```python
from build123d import *

# Parameters (mm, degrees)
SKETCH1_R           = 0.75
BOSS_EXTRUDE1_DEPTH = 1.2


with BuildPart() as part:
    # Sketch1 → Boss-Extrude1 (new body)
    with BuildSketch(Plane.XY):
        with BuildLine():
            Line((13, 8.65), (-13, 8.65))
            Line((-13, 8.65), (-13, 7.6))
            ThreePointArc((-13, 7.6), (-12.469669914, 7.380330086), (-12.25, 6.85))
            ThreePointArc((-12.25, 6.85), (-12.469669914, 6.319669914), (-13, 6.1))
            Line((-13, 6.1), (-13, 5.4))
            ThreePointArc((-13, 5.4), (-12.469669914, 5.180330086), (-12.25, 4.65))
            ThreePointArc((-12.25, 4.65), (-12.469669914, 4.119669914), (-13, 3.9))
            Line((-13, 3.9), (-13, -3.9))
            ThreePointArc((-13, -3.9), (-12.469669914, -4.119669914), (-12.25, -4.65))
            ThreePointArc((-12.25, -4.65), (-12.469669914, -5.180330086), (-13, -5.4))
            Line((-13, -5.4), (-13, -6.1))
            ThreePointArc((-13, -6.1), (-12.469669914, -6.319669914), (-12.25, -6.85))
            ThreePointArc((-12.25, -6.85), (-12.469669914, -7.380330086), (-13, -7.6))
            Line((-13, -7.6), (-13, -8.65))
            Line((-13, -8.65), (13, -8.65))
            Line((13, -8.65), (13, -7.6))
            ThreePointArc((13, -7.6), (12.25, -6.85), (13, -6.1))
            Line((13, -6.1), (13, -5.4))
            ThreePointArc((13, -5.4), (12.25, -4.65), (13, -3.9))
            Line((13, -3.9), (13, 3.9))
            ThreePointArc((13, 3.9), (12.25, 4.65), (13, 5.4))
            Line((13, 5.4), (13, 6.1))
            ThreePointArc((13, 6.1), (12.25, 6.85), (13, 7.6))
            Line((13, 7.6), (13, 8.65))
        make_face()
        with Locations((-11.3, -6.85)):
            Circle(SKETCH1_R, mode=Mode.SUBTRACT)
        with Locations((-11.3, -4.65)):
            Circle(SKETCH1_R, mode=Mode.SUBTRACT)
        with Locations((11.3, -6.85)):
            Circle(SKETCH1_R, mode=Mode.SUBTRACT)
        with Locations((11.3, -4.65)):
            Circle(SKETCH1_R, mode=Mode.SUBTRACT)
        with Locations((-11.3, 4.65)):
            Circle(SKETCH1_R, mode=Mode.SUBTRACT)
        with Locations((-11.3, 6.85)):
            Circle(SKETCH1_R, mode=Mode.SUBTRACT)
        with Locations((11.3, 4.65)):
            Circle(SKETCH1_R, mode=Mode.SUBTRACT)
        with Locations((11.3, 6.85)):
            Circle(SKETCH1_R, mode=Mode.SUBTRACT)
    extrude(amount=BOSS_EXTRUDE1_DEPTH)


solid = part.part
```
Source: CAD feature listing. Evaluate the final solid. Frame: model axes, mm. Round coordinates to 2 decimals unless told otherwise and drop trailing zeros. Write each loop counter-clockwise with the first axis right and the second up, starting at its lowest first coordinate (ties: lowest second). Pieces come first, ordered by that corner, then holes. Notation, with made-up numbers: M 72.5,6 L 125.5,6 A10 ccw 125.5,22 Z; hole C -25.75,67.25 d5. An arc over 180 degrees is marked long. Use CSV: the item, a comma, the result in double quotes. Start each with the question number.
Q1. Line query: line 1 (Y direction, x = -11.3, z = 0.6); line 2 (X direction, y = -6.25, z = 0.8); line 3 (Y direction, x = -11, z = 0.95). Output: solid intervals per line, ascending. Write a range as from..to.
Q2. Cut plane C-C on y = 5. Output: boundary loops of the cut face in (x, z).
Q3. Cut plane B-B on z = 0.5. Count the separate pieces of the cut face and the enclosed holes in it, plus the area to 3 significant figures.
Q4. Cut plane A-A on x = -11.3. Output: boundary loops of the cut face in (y, z).
Q5. Pull-direction query (X, two-part tool) for faces 1 (the face through (0, 0, 0)), 2 (the face through (-10.61, -4.94, 0.59)), 3 (the face through (12.25, 4.63, 0.59)); classes: +X half, -X half, draft (parallel to the pull), parting line (faces both ways), or undercut.
Q6. First-contact query: P1, Ø0.9, axis at x = -11.3, y = 6.85, coming from the +Z side. Flat tip, straight axial feed; report the tip coordinate or a pass-through.
Results found:
1,line 1,"-8.65..-7.6, -6.1..-5.4, -3.9..3.9, 5.4..6.1, 7.6..8.65"
1,line 2,"-12.55..-11.75, -10.85..10.85, 11.75..12.55"
1,line 3,"-8.65..-7.54, -6.16..-5.34, -3.96..3.96, 5.34..6.16, 7.54..8.65"
2,outline,"M -12.34,0 L -11.96,0 L -11.96,1.2 L -12.34,1.2 Z; M -10.64,0 L 10.64,0 L 10.64,1.2 L -10.64,1.2 Z; M 11.96,0 L 12.34,0 L 12.34,1.2 L 11.96,1.2 Z"
3,separate pieces,"1"
3,enclosed holes,"8"
3,area,"429 mm^2"
4,outline,"M -8.65,0 L -7.6,0 L -7.6,1.2 L -8.65,1.2 Z; M -6.1,0 L -5.4,0 L -5.4,1.2 L -6.1,1.2 Z; M -3.9,0 L 3.9,0 L 3.9,1.2 L -3.9,1.2 Z; M 5.4,0 L 6.1,0 L 6.1,1.2 L 5.4,1.2 Z; M 7.6,0 L 8.65,0 L 8.65,1.2 L 7.6,1.2 Z"
5,face 1,"draft"
5,face 2,"undercut"
5,face 3,"+X half"
6,P1,"through"
